Part model, mm, in its own coordinate system. A direction names the side the tool comes from. Coordinates: 2 decimals unless noted, no trailing zeros. Loops run counter-clockwise (first coordinate to the right, second up) from the corner with the lowest first, then second, coordinate; pieces in that order, holes last. Notation, with made-up numbers: M 87.5,-30.75 L 103.5,-30.75 A18 cw 103.5,-4.75 Z; hole C 1,72 d4. An arc over 180 degrees is marked long. Use a Markdown table: item, result. Add a question column.
1) Pull direction Z, two halves, no side cores. Call faces 1 (the flat face through (46.565, 4, 13)), 2 (the cylindrical face through (59.925, 21.632, 178.815)), 3 (the flat face through (39, -1, 215)): released by +Z, released by -Z, zero draft, split by the parting line, or undercut.
2) Wall check: probe 1 along Y at (x, z) = (-16.5, 169.5); probe 2 along Z at (x, y) = (56, -3); probe 3 along X at (y, z) = (17.5, 102). Give the ranges that are in metal, low to high. Write a range as from..to.
3) Band-saw the part on B-B (x = 14). List the corners of the cut face in (y, z), plus the area to 3 significant figures.
4) Band-saw the part on C-C (z = 175). List the corners of the cut face in (x, y).
5) Band-saw the part on D-D (x = 48.5). List the corners of the cut face in (y, z).
6) Pin check, flat tips, straight feed: pin 1 Ø1.4 at (x, z) = (38, 17) entering from +Y; pin 2 Ø2 at (x, y) = (45.5, 3) entering from -Z. Stop position of each tip, or through.
7) Tool access for faces 4 (the flat face through (70.724, -1, 96)), 5 (the flat face through (20, -22.37, 96)), 6 (the cylindrical face through (34.523, 2.867, 204.86)), 7 (the flat face through (43.982, 4, 13)), 8 (the cylindrical face through (-21.18, 21.63, 19.13)): list every direction of +Z, -Z, +X, -X, +Y, -Y with a clear straight run to the whole face (end or side of a thin tool).
8) Band-saw the part on A-A (y = -13). List the corners of the cut face in (x, z), plus the area to 3 significant figures.
from build123d import *

# Parameters (mm, degrees)
SKETCH1_W           = 100
SKETCH1_H           = 42.77
BOSS_EXTRUDE1_DEPTH = 195
SKETCH2_R           = 4
BOSS_EXTRUDE2_DEPTH = 2.5
FILLET1_R           = 3
SKETCH3_R           = 5.7
BOSS_EXTRUDE3_DEPTH = 20
CUT_EXTRUDE1_DEPTH  = 23
SKETCH5_W           = 2.767644168
SKETCH5_H           = 5.042715582
SKETCH5_W_2         = 2.583134557
SKETCH5_H_2         = 3.628689021
BOSS_EXTRUDE4_DEPTH = 20
SKETCH6_W           = 2.767644168
SKETCH6_H           = 5.042715582
BOSS_EXTRUDE5_DEPTH = 3


with BuildPart() as part:
    # Sketch1 → Boss-Extrude1 (new body)
    with BuildSketch(Plane.XY):
        with Locations((20.723910559, -0.985431434)):
            Rectangle(SKETCH1_W, SKETCH1_H)
    extrude(amount=BOSS_EXTRUDE1_DEPTH)

    # Sketch2 → Boss-Extrude2 (add)
    with BuildSketch(Plane(origin=(0, 20.399568566, 0), x_dir=(1, 0, 0), z_dir=(0, 1, 0))):
        with BuildLine():
            ThreePointArc((62.723910559, -20), (61.552337684, -17.171572875), (58.723910559, -16))
            Line((58.723910559, -16), (58.723910559, -20))
            Line((58.723910559, -20), (62.723910559, -20))
        make_face()
        with BuildLine():
            Line((58.723910559, -20), (58.723910559, -16))
            ThreePointArc((58.723910559, -16), (55.895483435, -22.828427125), (62.723910559, -20))
            Line((62.723910559, -20), (58.723910559, -20))
        make_face()
        with Locations(Location((-17.276089441, -20, 0), (0, 0, 270))):
            Circle(SKETCH2_R)
        with Locations(Location((-17.276089441, -175, 0), (0, 0, 90))):
            Circle(SKETCH2_R)
        with Locations(Location((58.723910559, -175, 0), (0, 0, 270))):
            Circle(SKETCH2_R)
    extrude(amount=BOSS_EXTRUDE2_DEPTH)

    # Fillet1
    fillet1_edges = [part.edges().sort_by_distance(p)[0] for p in [
        (70.723910559, -0.985431434, 195),
        (20.723910559, 20.399568566, 195),
        (-29.276089441, -0.985431434, 195),
        (20.723910559, 20.399568566, 0),
        (70.723910559, -0.985431434, 0),
        (20.723910559, -22.370431434, 0),
        (-29.276089441, -0.985431434, 0),
        (20.723910559, -22.370431434, 195),
        (-29.276089441, 20.399568566, 97.5),
        (70.723910559, 20.399568566, 97.5),
        (70.723910559, -22.370431434, 97.5),
        (-29.276089441, -22.370431434, 97.5),
    ]]
    fillet(fillet1_edges, radius=FILLET1_R)

    # Sketch3 → Boss-Extrude3 (add)
    with BuildSketch(Plane.XY.offset(195)):
        with Locations((38.723910559, -0.985431434)):
            Circle(SKETCH3_R)
    extrude(amount=BOSS_EXTRUDE3_DEPTH)

    # Sketch4 → Cut-Extrude1 (cut)
    with BuildSketch(Plane(origin=(0, 0, 0), x_dir=(-1, 0, 0), z_dir=(0, 0, -1))):
        Polygon((-50.723910559, 0), (-50.723910559, -3), (-45.097599839, -8.62631072), (-31.35022128, -8.62631072), (-25.723910559, -3), (-25.723910559, 9), (-50.723910559, 9), align=None)
    extrude(amount=-CUT_EXTRUDE1_DEPTH, mode=Mode.SUBTRACT)

    # Sketch5 → Boss-Extrude4 (add)
    with BuildSketch(Plane(origin=(0, 0, 23), x_dir=(-1, 0, 0), z_dir=(0, 0, -1))):
        with Locations((-37.98516428, -2.521357791)):
            Rectangle(SKETCH5_W, SKETCH5_H)
        with Locations((-45.273293924, 3.598484544)):
            Rectangle(SKETCH5_W_2, SKETCH5_H_2)
        with Locations((-30.697034638, 3.598484544)):
            Rectangle(SKETCH5_W_2, SKETCH5_H_2)
    extrude(amount=BOSS_EXTRUDE4_DEPTH)

    # Sketch6 → Boss-Extrude5 (add)
    with BuildSketch(Plane(origin=(0, 0, 3), x_dir=(-1, 0, 0), z_dir=(0, 0, -1))):
        with Locations((-37.98516428, -2.521357791)):
            Rectangle(SKETCH6_W, SKETCH6_H)
    extrude(amount=BOSS_EXTRUDE5_DEPTH)


solid = part.part
Entries:
| question | item | result |
|---|---|---|
| 1 | face 1 | zero draft |
| 1 | face 2 | undercut |
| 1 | face 3 | released by +Z |
| 2 | probe 1 | -22.37..20.4 |
| 2 | probe 2 | 0..195 |
| 2 | probe 3 | -29.27..70.72 |
| 3 | outline | M -22.37,3 A3 ccw -19.37,0 L 17.4,0 A3 ccw 20.4,3 L 20.4,192 A3 ccw 17.4,195 L -19.37,195 A3 ccw -22.37,192 Z |
| 3 | area | 8,330 mm2 |
| 4 | outline | M -29.28,-19.37 A3 ccw -26.28,-22.37 L 67.72,-22.37 A3 ccw 70.72,-19.37 L 70.72,17.4 A3 ccw 67.72,20.4 L 62.72,20.4 L 62.72,22.9 L 54.72,22.9 L 54.72,20.4 L -13.28,20.4 L -13.28,22.9 L -21.28,22.9 L -21.28,20.4 L -26.28,20.4 A3 ccw -29.28,17.4 Z |
| 5 | outline | M -22.37,3 A3 ccw -19.37,0 L -5.22,0 L -5.22,23 L 9,23 L 9,0 L 17.4,0 A3 ccw 20.4,3 L 20.4,192 A3 ccw 17.4,195 L -19.37,195 A3 ccw -22.37,192 Z |
| 6 | pin 1 | y = 20.4 |
| 6 | pin 2 | z = 3 |
| 7 | face 4 | +Z, -Z, +X, +Y, -Y |
| 7 | face 5 | +Z, -Z, +X, -X, -Y |
| 7 | face 6 | +Z |
| 7 | face 7 | -Z |
| 7 | face 8 | +Y |
| 8 | outline | M -29.28,3 A3 ccw -26.28,0 L 67.72,0 A3 ccw 70.72,3 L 70.72,192 A3 ccw 67.72,195 L -26.28,195 A3 ccw -29.28,192 Z |
| 8 | area | 19,500 mm2 |
